from build123d import *

# Parameters (mm, degrees)
F0_W          = 10
F0_H          = 20
F0_W_2        = 8
F0_H_2        = 18
F1_DEPTH      = 10
F2_W          = 2
F2_H          = 16
F3_DEPTH      = 10
F3_DEPTH_BACK = 0.01


with BuildPart() as f1:
    # F0 (on Front) → F1 (new body)
    with BuildSketch(Plane.XZ):
        with Locations((4, 9)):
            Rectangle(F0_W, F0_H)
        with Locations((4, 9)):
            Rectangle(F0_W_2, F0_H_2, mode=Mode.SUBTRACT)
    extrude(amount=F1_DEPTH)

    # F2 (on face) → F3 (join, two sides)
    with BuildSketch(Plane(origin=(-1, 0, 0), x_dir=(0, -1, 0), z_dir=(-1, 0, 0))) as f3_sk:
        with Locations((2.5, 9)):
            Rectangle(F2_W, F2_H)
    extrude(amount=-F3_DEPTH)
    extrude(f3_sk.sketch, amount=F3_DEPTH_BACK)


solid = f1.part
Geometry check sheet. Reference: the model listing, model coordinates, mm. A direction names the side the tool comes from. Give positions to 0.01 mm unless a question says otherwise; leave off trailing zeros. Write each loop counter-clockwise with the first axis right and the second up, starting at its lowest first coordinate (ties: lowest second). Pieces come first, ordered by that corner, then holes. Notation, with made-up numbers: M 71,-11 L 90,-11 A26 ccw 90,27 Z; hole C 36,-16.75 d2. An arc over 180 degrees is marked long. Answer as CSV lines item,"result". Start each with the question number.
Q1. Release check for a two-part mould opening along X. For faces 6 (the face through (-1, -6, 9)), 7 (the face through (4, -5, -1)), 8 (the face through (9, -5, 9)), 9 (the face through (4, -2, 1)) record: pulls with the +X half, pulls with the -X half, needs draft (parallel to the pull), parting line crosses it, or undercut.
Q2. Material ranges on L1, parallel to Z at x = 5.75, y = -2.75; L2, parallel to X at y = -4, z = 7; L3, parallel to Z at x = 5.25, y = -1.25, recorded low to high.
Q3. Section check A-A, the plane y = -1.75. Give the number of separate pieces and of enclosed holes in the cut face, then the cut area to 3 significant figures.
Q4. Section check B-B, the plane x = 0.75. Record the cut outline in (y, z), then the cut area to 3 significant figures.
Q5. Tool access check on faces 1 (the face through (4, -5, 18)), 2 (the face through (8, -6, 9)), 3 (the face through (4, -1.5, 9)), 4 (the face through (4, -3.5, 9)), 5 (the face through (-0.5, 0, 9.8)). Record the directions out of +Z, -Z, +X, -X, +Y, -Y that give a thin tool (end or side, any length) a straight path to the whole face; none if there is none.
Q6. Go/stop test with flat-tipped pins: pin 1 (3 mm diameter, centred on y = -6.5, z = 9, fed in from -X); pin 2 (3 mm diameter, centred on x = 5.5, z = 10.5, fed in from +Y); pin 3 (4 mm diameter, centred on x = 4, z = 5.5, fed in from -Y). Record where each tip stops, or that it passes through.
Geometry says:
1,face 6,"pulls with the -X half"
1,face 7,"needs draft"
1,face 8,"pulls with the +X half"
1,face 9,"undercut"
2,L1,"-1 to 0, 1 to 17, 18 to 19"
2,L2,"-1 to 0, 8 to 9"
2,L3,"-1 to 0, 18 to 19"
3,separate pieces,"1"
3,enclosed holes,"2"
3,area,"184 mm^2"
4,outline,"M -10,-1 L 0,-1 L 0,0 L -10,0 Z; M -10,18 L 0,18 L 0,19 L -10,19 Z; M -3.5,1 L -1.5,1 L -1.5,17 L -3.5,17 Z"
4,area,"52.0 mm^2"
5,face 1,"+Y, -Y"
5,face 2,"none"
5,face 3,"+Y"
5,face 4,"-Y"
5,face 5,"+Z, -Z, +X, -X, +Y"
6,pin 1,"x = -1"
6,pin 2,"y = -1.5"
6,pin 3,"y = -3.5"
